The model under review builds one solid part; all positions refer to its coordinate system, in mm. A direction names the side the tool comes from. Give positions to 0.01 mm unless a question says otherwise; leave off trailing zeros. Write each loop counter-clockwise with the first axis right and the second up, starting at its lowest first coordinate (ties: lowest second). Pieces come first, ordered by that corner, then holes. Notation, with made-up numbers: (-26, -28.75) - (25, -28.75) arc R29 ccw to (25, -1.75) - close; hole circle Ø9 at (6.5, 76.25). An arc over 180 degrees is marked (long way). One line per question, with ' | ' between items. Start each with the question number.
```python
from build123d import *

# Parameters (mm, degrees)
BOSS_EXTRUDE1_DEPTH = 67
SKETCH2_R           = 2.15
SKETCH2_R_2         = 19.1
CUT_EXTRUDE1_DEPTH  = 67
SKETCH3_W           = 70
SKETCH3_H           = 4.9
BOSS_EXTRUDE2_DEPTH = 63
SKETCH4_W           = 20
SKETCH4_H           = 67
BOSS_EXTRUDE3_DEPTH = 10
CHAMFER1_SIZE       = 80
CHAMFER1_SIZE_2     = 50
SKETCH6_W           = 80
SKETCH6_H           = 30
CUT_EXTRUDE2_DEPTH  = 13
SKETCH7_R           = 2.15
CUT_EXTRUDE3_DEPTH  = 100
CUT_EXTRUDE4_DEPTH  = 100
FILLET2_R           = 8
SKETCH9_W           = 7.2
SKETCH9_H           = 3.5
CUT_EXTRUDE5_DEPTH  = 14
CHAMFER2_SIZE       = 2
CHAMFER3_SIZE       = 2
CHAMFER4_SIZE       = 0.8
CHAMFER5_SIZE       = 3


with BuildPart() as part:
    # Sketch1 → Boss-Extrude1 (new body)
    with BuildSketch(Plane(origin=(0, 0, 0), x_dir=(1, 0, 0), z_dir=(0, 1, 0))):
        Polygon((0, 0), (0, 90), (7, 90), (7, 20), (70, 20), (70, 0), align=None)
    extrude(amount=BOSS_EXTRUDE1_DEPTH)

    # Sketch2 → Cut-Extrude1 (cut)
    with BuildSketch(Plane(origin=(7, 0, 0), x_dir=(0, 0, -1), z_dir=(1, 0, 0))):
        with Locations((83.57, 57.07)):
            Circle(SKETCH2_R)
        with Locations((36.43, 57.07)):
            Circle(SKETCH2_R)
        with Locations((36.43, 9.93)):
            Circle(SKETCH2_R)
        with Locations((83.57, 9.93)):
            Circle(SKETCH2_R)
        with Locations((60, 33.5)):
            Circle(SKETCH2_R_2)
    extrude(amount=-CUT_EXTRUDE1_DEPTH, mode=Mode.SUBTRACT)

    # Sketch3 → Boss-Extrude2 (add)
    with BuildSketch(Plane(origin=(7, 0, 0), x_dir=(0, 0, -1), z_dir=(1, 0, 0))):
        with Locations((55, 64.55)):
            Rectangle(SKETCH3_W, SKETCH3_H)
        with Locations((55, 2.45)):
            Rectangle(SKETCH3_W, SKETCH3_H)
    extrude(amount=BOSS_EXTRUDE2_DEPTH)

    # Sketch4 → Boss-Extrude3 (add)
    with BuildSketch(Plane(origin=(70, 0, 0), x_dir=(0, 0, -1), z_dir=(1, 0, 0))):
        with Locations((10, 33.5)):
            Rectangle(SKETCH4_W, SKETCH4_H)
    extrude(amount=BOSS_EXTRUDE3_DEPTH)

    # Chamfer1
    # the kernel refuses this chamfer: 80, 50 mm, written as the material it takes off along each edge
    with BuildSketch(Plane(origin=(70, -206.827451207, -90), x_dir=(0.020500139102813345, 0, 0.9997898500668855), z_dir=(0, 1, 0))) as chamfer1_piece_1_section:
        Polygon((CHAMFER1_SIZE * 0.999789850067, -CHAMFER1_SIZE * 0.0205001391028), (-CHAMFER1_SIZE_2 * 0.0205001391028, -CHAMFER1_SIZE_2 * 0.999789850067), (0, 0), align=None)
    chamfer1_piece_1 = extrude(amount=418.554902414, mode=Mode.PRIVATE)
    chamfer1_piece_1 = split(chamfer1_piece_1, bisect_by=Plane(origin=(53.400446445, 2.45, -20), z_dir=(0, 0, -1)), keep=Keep.TOP, mode=Mode.PRIVATE)
    add(chamfer1_piece_1, mode=Mode.SUBTRACT)
    with BuildSketch(Plane(origin=(70, 273.827451207, -90), x_dir=(0.020500139102813345, 0, 0.9997898500668855), z_dir=(0, -1, 0))) as chamfer1_piece_2_section:
        Polygon((CHAMFER1_SIZE * 0.999789850067, CHAMFER1_SIZE * 0.0205001391028), (-CHAMFER1_SIZE_2 * 0.0205001391028, CHAMFER1_SIZE_2 * 0.999789850067), (0, 0), align=None)
    chamfer1_piece_2 = extrude(amount=418.554902414, mode=Mode.PRIVATE)
    chamfer1_piece_2 = split(chamfer1_piece_2, bisect_by=Plane(origin=(53.400446445, 64.55, -20), z_dir=(0, 0, -1)), keep=Keep.TOP, mode=Mode.PRIVATE)
    add(chamfer1_piece_2, mode=Mode.SUBTRACT)

    # Sketch6 → Cut-Extrude2 (cut)
    with BuildSketch(Plane.XY):
        with Locations((40, 33.5)):
            Rectangle(SKETCH6_W, SKETCH6_H)
    extrude(amount=-CUT_EXTRUDE2_DEPTH, mode=Mode.SUBTRACT)

    # Sketch7 → Cut-Extrude3 (cut)
    with BuildSketch(Plane(origin=(0, 67, 0), x_dir=(1, 0, 0), z_dir=(0, 1, 0))):
        with Locations(Location((15, 8, 0), (0, 0, 270))):
            Circle(SKETCH7_R)
        with Locations(Location((65, 8, 0), (0, 0, 270))):
            Circle(SKETCH7_R)
    extrude(amount=-CUT_EXTRUDE3_DEPTH, mode=Mode.SUBTRACT)

    # Sketch8 → Cut-Extrude4 (cut)
    with BuildSketch(Plane(origin=(0, 0, -20), x_dir=(-1, 0, 0), z_dir=(0, 0, -1))):
        with BuildLine():
            Line((-63.5, 35.7), (-23.5, 35.7))
            ThreePointArc((-23.5, 35.7), (-21.3, 33.5), (-23.5, 31.3))
            Line((-23.5, 31.3), (-63.5, 31.3))
            ThreePointArc((-63.5, 31.3), (-65.7, 33.5), (-63.5, 35.7))
        make_face()
    extrude(amount=-CUT_EXTRUDE4_DEPTH, mode=Mode.SUBTRACT)

    # Fillet2
    fillet2_edges = [part.edges().sort_by_distance(p)[0] for p in [
        (7, 33.5, -20),
    ]]
    fillet(fillet2_edges, radius=FILLET2_R)

    # Sketch9 → Cut-Extrude5 (cut)
    with BuildSketch(Plane.XY):
        with Locations((65, 57.75)):
            Rectangle(SKETCH9_W, SKETCH9_H)
        with Locations((15, 57.75)):
            Rectangle(SKETCH9_W, SKETCH9_H)
        with Locations((65, 9.25)):
            Rectangle(SKETCH9_W, SKETCH9_H)
        with Locations((15, 9.25)):
            Rectangle(SKETCH9_W, SKETCH9_H)
    extrude(amount=-CUT_EXTRUDE5_DEPTH, mode=Mode.SUBTRACT)

    # Chamfer2
    chamfer2_edges = [part.edges().sort_by_distance(p)[0] for p in [
        (80, 48.5, -6.5),
        (80, 18.5, -6.5),
        (0, 18.5, -6.5),
        (0, 48.5, -6.5),
    ]]
    chamfer(chamfer2_edges, length=CHAMFER2_SIZE)

    # Chamfer3
    chamfer3_edges = [part.edges().sort_by_distance(p)[0] for p in [
        (80, 58.75, 0),
        (80, 8.25, 0),
        (0, 58.75, 0),
        (0, 8.25, 0),
    ]]
    chamfer(chamfer3_edges, length=CHAMFER3_SIZE)

    # Chamfer4
    chamfer4_edges = [part.edges().sort_by_distance(p)[0] for p in [
        (40, 18.5, 0),
        (40, 48.5, 0),
    ]]
    chamfer(chamfer4_edges, length=CHAMFER4_SIZE)

    # Chamfer5
    chamfer5_edges = [part.edges().sort_by_distance(p)[0] for p in [
        (0, 33.5, -40.9),
    ]]
    chamfer(chamfer5_edges, length=CHAMFER5_SIZE)


solid = part.part
```
Item 1: Take a section at D-D (z = -60). Give the boundary of the cut face in (x, y).
Item 2: Take a section at C-C (z = -83.57). Give the boundary of the cut face in (x, y), plus the area to 3 significant figures.
Item 3: Take a section at A-A (y = 33.5). Give the boundary of the cut face in (x, z).
Item 4: The part is to be moulded in two halves that separate along Y. For faces 1 (the flat face through (18.6, 9, -7)), 2 (the flat face through (31, 0, -34)), 3 (the cylindrical face through (13.09, 14.8, -7.01)), say which applies: +Y half, -Y half, draft (parallel to the pull), parting line (faces both ways), or undercut.
Item 5: For probe 1 along Y at (x, z) = (63.5, -12.5); probe 2 along X at (y, z) = (5, -8); probe 3 along Y at (x, z) = (15.5, -63), list the stretches that pass through material, from the lowest coordinate up.
Item 6: Machinability: for faces 4 (the cylindrical face through (65.7, 33.5, -16.5)), 5 (the flat face through (65, 7.5, -5)), 6 (the cylindrical face through (3.549, 9.107, -85.556)), 7 (the flat face through (39, 48.5, -7)), 8 (the flat face through (29, 62.1, -47)), which of the approach directions +Z, -Z, +X, -X, +Y, -Y give a long, thin tool a straight path to every point of the face, cutting with its end or side? Answer none if there is none.
Item 7: Clearance check with flat-ended pins moving along their axes: P1, Ø6, axis at x = 31.5, z = -36.5, coming from the -Y side; P2, Ø1.5, axis at x = 8.5, y = 46, coming from the -Z side; P3, Ø12, axis at x = 54.5, y = 13.5, coming from the -Z side; P4, Ø5.5, axis at y = 57.07, z = -36.43, coming from the +X side. State where each tip first meets the part, or that it passes through.
Item 8: Take a section at B-B (x = 29). Give the boundary of the cut face in (y, z).
Check sheet entries:
1) outline: (0, 0) - (38.75, 0) - (38.75, 4.9) - (7, 4.9) - (7, 14.4) - (3, 14.4) - (0, 11.4) - close; (0, 55.6) - (3, 52.6) - (7, 52.6) - (7, 62.1) - (38.75, 62.1) - (38.75, 67) - (0, 67) - close
2) outline: (0, 0) - (24.02, 0) - (24.02, 4.9) - (7, 4.9) - (7, 7.78) - (0, 7.78) - close; (0, 12.08) - (7, 12.08) - (7, 54.92) - (0, 54.92) - close; (0, 59.22) - (7, 59.22) - (7, 62.1) - (24.02, 62.1) - (24.02, 67) - (0, 67) - close | area: 576 mm^2
3) outline: (0, -90) - (7, -90) - (7, -79.1) - (3, -79.1) - (0, -82.1) - close; (0, -37.9) - (3, -40.9) - (7, -40.9) - (7, -28) arc R8 cw to (15, -20) - (21.3, -20) - (21.3, -13) - (0, -13) - close; (65.7, -20) - (80, -20) - (80, -13) - (65.7, -13) - close
4) face 1: undercut | face 2: -Y half | face 3: draft
5) probe 1: y = 0 to 7.5, 11 to 18.5, 48.5 to 56, 59.5 to 67 | probe 2: x = 0 to 12.85, 17.15 to 62.85, 67.15 to 80 | probe 3: y = 0 to 4.9, 62.1 to 67
6) face 4: +Z, -Z | face 5: +Z | face 6: +X, -X | face 7: +Z, +X, -X | face 8: -Z, +X
7) P1: stops at y = 0 | P2: stops at z = -24.62 | P3: stops at z = -20 | P4: stops at x = 7
8) outline: (0, -75.6) - (4.9, -75.6) - (4.9, -20) - (31.3, -20) - (31.3, -13) - (18.5, -13) - (18.5, -0.8) - (17.7, 0) - (0, 0) - close; (35.7, -20) - (62.1, -20) - (62.1, -75.6) - (67, -75.6) - (67, 0) - (49.3, 0) - (48.5, -0.8) - (48.5, -13) - (35.7, -13) - close
